Here's how the part is built. I have some questions about the finished solid (model axes, mm). A direction names the side the tool comes from. Give positions to 0.01 mm unless a question says otherwise; leave off trailing zeros. Loops run counter-clockwise (first coordinate to the right, second up) from the corner with the lowest first, then second, coordinate; pieces in that order, holes last. Notation, with made-up numbers: (10.5, 4) - (15.5, 4) arc R17 ccw to (15.5, 8) - close; hole circle Ø7 at (-11, 67.25). An arc over 180 degrees is marked (long way). Use a Markdown table: item, result.
Autodesk Inventor part; units mm, degrees
ref_plane "YZ Plane" through (0, 0, 0) normal (1, 0, 0) x (0, 1, 0)
ref_plane "XZ Plane" through (0, 0, 0) normal (0, 1, 0) x (-1, 0, 0)
ref_plane "XY Plane" through (0, 0, 0) normal (0, 0, 1) x (1, 0, 0)
sketch "Sketch1" plane through (0, 0, 0) normal (0, 1, 0) x (-1, 0, 0)
  line L0 (-2.8391, 8.5286) -> (6.6609, 8.5286)
  line L1 (6.6609, 8.5286) -> (6.6609, -5.4714)
  line L2 (-2.8391, 8.5286) -> (-2.8391, -5.4714)
  line L3 (-2.8391, -5.4714) -> (6.6609, -5.4714)
  line L4 (-0.3391, 8.5286) -> (-0.3391, -5.4714)
  line L5 (4.1609, 8.5286) -> (4.1609, -5.4714)
  line L6 (-2.8391, 8.5286) -> (-8.0891, 8.5286)
  line L7 (-8.0891, 8.5286) -> (-8.0891, -5.4714)
  line L8 (-8.0891, -5.4714) -> (-2.8391, -5.4714)
  line L9 (6.6609, 8.5286) -> (11.9109, 8.5286)
  line L10 (11.9109, 8.5286) -> (11.9109, -5.4714)
  line L11 (11.9109, -5.4714) -> (6.6609, -5.4714)
  circle A0 centre (-5.4641, 1.5286) radius 1.5
  circle A1 centre (9.2859, 1.5286) radius 1.5
  point P0 (0, 0)
  dimension "d0" = 4.5
  dimension "d3" = 2.5
  dimension "d5" = 2.5
  dimension "d7" = 20
  dimension "d8" = 5.25
  dimension "d9" = 5.25
  dimension "d10" = 14
  dimension "d11" = 3
  dimension "d12" = 3
  dimension "d27" = 2.625
  dimension "d28" = 2.625
extrude "Extrusion1" add sketch "Sketch1" along normal blind 2
sketch "Sketch2" plane through (0, 2, 0) normal (0, 1, 0) x (1, 0, 0)
  line L0 (8.0891, 5.4714) -> (-11.9109, 5.4714)
  line L1 (-11.9109, -8.5286) -> (8.0891, -8.5286)
  line L2 (-4.1609, 5.4714) -> (-4.1609, -8.5286)
  line L3 (-4.1609, -8.5286) -> (0.3391, -8.5286)
  line L4 (0.3391, -8.5286) -> (0.3391, 5.4714)
  line L5 (0.3391, 5.4714) -> (2.8391, 5.4714)
  line L6 (2.8391, 5.4714) -> (2.8391, -8.5286)
  line L7 (-6.6609, 5.4714) -> (-6.6609, -8.5286)
  circle A0 centre (5.4641, -1.5286) radius 1.5
  point P0 (0, 0)
  dimension "d16" = 4.5
  dimension "d17" = 2.5
  dimension "d18" = 2.5
  dimension "d29" = 2.625
extrude "Extrusion2" add sketch "Sketch2" along normal blind 8 contours L6 L1 L4 L0 | L2 L1 L7 L0
fillet "Fillet1" radius 5 4 edges at (-5.4109, 10, -5.4714) (-5.4109, 10, 8.5286) (1.5891, 10, 8.5286) (1.5891, 10, -5.4714)
sketch "Sketch3" plane through (-6.6609, 2, -5.4714) normal (-1, 0, 0) x (0, 0, 1)
  line L0 (14, 0) -> (0, 0)
  circle A0 centre (7, 5) radius 1.5
  point P0 (5.4714, -2)
  dimension "d23" = 3
  dimension "d24" = 5
extrude "Extrusion3" cut sketch "Sketch3" against normal blind 20
properties material "ABS Plastic"
(1) Suppose I cut it at D-D on z = 5.5. Write out the boundary of the cut face in (x, y).
A:
| item | result |
|---|---|
| outline | (-11.91, 0) - (8.09, 0) - (8.09, 2) - (2.84, 2) - (2.84, 9.59) - (0.34, 9.59) - (0.34, 2) - (-4.16, 2) - (-4.16, 9.59) - (-6.66, 9.59) - (-6.66, 2) - (-11.91, 2) - close |
(2) Suppose I cut it at B-B on x = -10.5. Write out the boundary of the cut face in (y, z), plus the area to 3 significant figures.
A:
| item | result |
|---|---|
| outline | (0, -5.47) - (2, -5.47) - (2, 0.65) - (0, 0.65) - close; (0, 2.41) - (2, 2.41) - (2, 8.53) - (0, 8.53) - close |
| area | 24.5 mm2 |
(3) Suppose I cut it at C-C on y = 7. Write out the boundary of the cut face in (x, z), plus the area to 3 significant figures.
A:
| item | result |
|---|---|
| outline | (-6.66, -5.05) - (-4.16, -5.05) - (-4.16, 0.03) - (-6.66, 0.03) - close; (-6.66, 3.03) - (-4.16, 3.03) - (-4.16, 8.11) - (-6.66, 8.11) - close; (0.34, -5.05) - (2.84, -5.05) - (2.84, 0.03) - (0.34, 0.03) - close; (0.34, 3.03) - (2.84, 3.03) - (2.84, 8.11) - (0.34, 8.11) - close |
| area | 50.8 mm2 |
(4) If I drill on line 1 (X direction, y = 2.5, z = 4.5); line 2 (Y direction, x = 6.75, z = 7.75), over which ranges is the centre line in solid material (lowest first)?
A:
| item | result |
|---|---|
| line 1 | -6.66 to -4.16, 0.34 to 2.84 |
| line 2 | 0 to 2 |
(5) Will these pins go through, and if not, where does the flat tip stop? pin 1 (6 mm diameter, centred on y = 9, z = 3.5, fed in from -X); pin 2 (5 mm diameter, centred on y = 7, z = 1.53, fed in from +X); pin 3 (2.5 mm diameter, centred on x = -8, z = 1.5, fed in from +Y); pin 4 (2.5 mm diameter, centred on y = 7, z = 1.53, fed in from -X).
A:
| item | result |
|---|---|
| pin 1 | x = -6.66 |
| pin 2 | x = 2.84 |
| pin 3 | y = 2 |
| pin 4 | through |
(6) We'd pull the mould along Z, two halves only. Please class faces 1 (the face through (4.078, 0.986, 2.103)), 2 (the face through (2.839, 5, 1)), 3 (the face through (-5.43, 8.57, -3.97)): pulls with the +Z half, pulls with the -Z half, needs draft (parallel to the pull), parting line crosses it, or undercut.
A:
| item | result |
|---|---|
| face 1 | undercut |
| face 2 | needs draft |
| face 3 | pulls with the -Z half |
(7) Suppose I cut it at A-A on y = 5.25. Write out the boundary of the cut face in (x, z), plus the area to 3 significant figures.
A:
| item | result |
|---|---|
| outline | (-6.66, -5.47) - (-4.16, -5.47) - (-4.16, 8.52) - (-6.66, 8.52) - close; (0.34, -5.47) - (2.84, -5.47) - (2.84, 8.52) - (0.34, 8.52) - close |
| area | 69.9 mm2 |
(8) On a 3-axis mill with a long thin cutter (end or side, diameter ignored), from which of +Z, -Z, +X, -X, +Y, -Y can I reach the whole of each face in a straight line? I mean faces 4 (the face through (5.5, 2, 3.2)), 5 (the face through (-2, 2, 2)), 6 (the face through (1.572, 5.536, 1.203)), 7 (the face through (-9.2, 2, 3.2)). Say none if no direction works.
A:
| item | result |
|---|---|
| face 4 | +Z, -Z, +X, +Y |
| face 5 | +Z, -Z, +Y |
| face 6 | +X, -X |
| face 7 | +Z, -Z, -X, +Y |
